Part print with two shaded views. Sizes in mm from the minimum x, y, z corner. A direction names the side the tool comes from. Give positions to 0.01 mm unless a question says otherwise; leave off trailing zeros. Write each loop counter-clockwise with the first axis right and the second up, starting at its lowest first coordinate (ties: lowest second). Pieces come first, ordered by that corner, then holes.
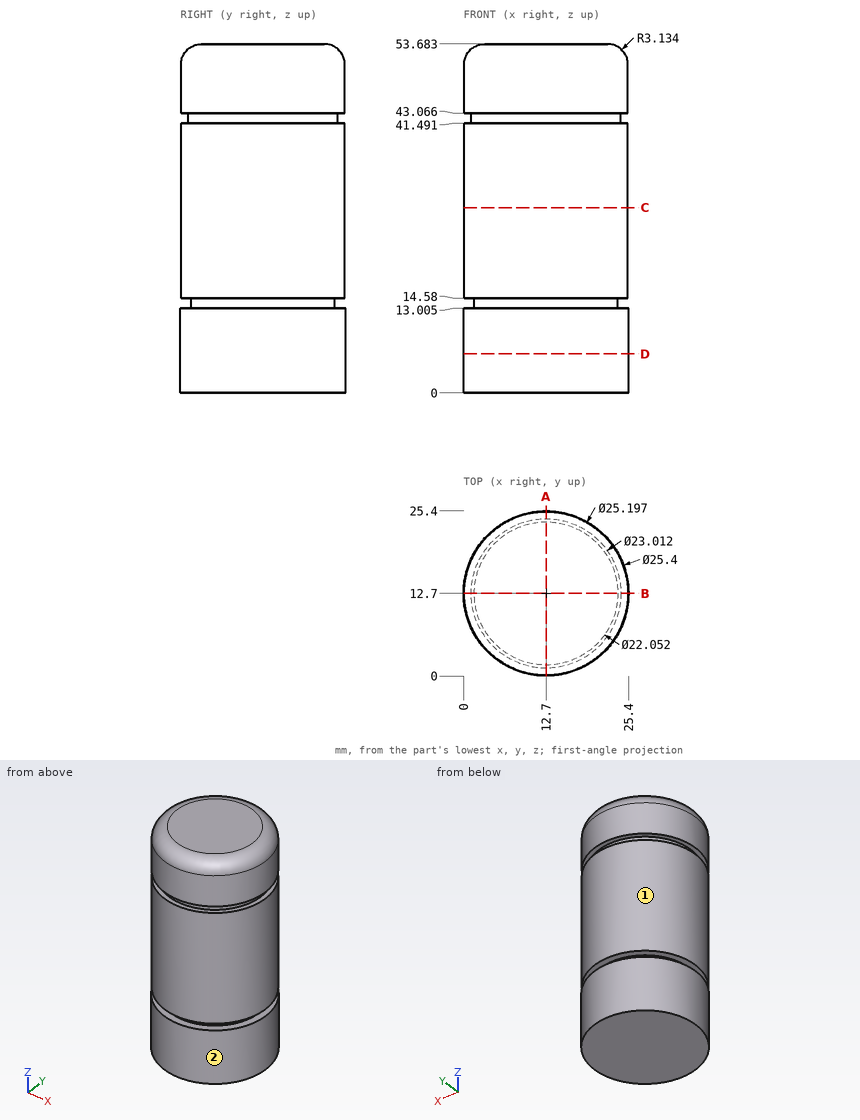
1) Wall check: L1, parallel to Z at x = 22.75, y = 19.5 (1 decimal); L2, parallel to Z at x = 12.5, y = 1 (1 decimal); L3, parallel to Z at x = 21.75, y = 16. Give the ranges that are in metal, low to high.
Answers follow:
L1: z = 0 to 13, 14.6 to 41.5, 43.1 to 52.2
L2: z = 0 to 13, 14.6 to 41.5, 43.1 to 52.7
L3: z = 0 to 53.68
2) Saw through at D-D, the plane z = 6. Write the cut outline in (x, y).
Answers follow:
outline: circle Ø25.4 at (12.7, 12.7)
3) 3-axis set-ups, long thin cutter, end or side, ignore diameter. For the marked faces 1 and 2: which of +Z, -Z, +X, -X, +Y, -Y reach the whole face in a straight line?
Answers follow:
face 1: +Z
face 2: +Z, -Z
4) Pin check, flat tips, straight feed: pin 1 Ø2 at (x, z) = (17.5, 10.5) entering from +Y; pin 2 Ø1.5 at (y, z) = (13.5, 14.5) entering from +X; pin 3 Ø2 at (y, z) = (6, 19.5) entering from +X (1 decimal). Stop position of each tip, or through.
Answers follow:
pin 1: stops at y = 24.82
pin 2: stops at x = 25.3
pin 3: stops at x = 23.9
5) Saw through at A-A, the plane x = 12.7. Write the cut outline in (y, z) (1 decimal).
Answers follow:
outline: (0, 0) - (25.4, 0) - (25.4, 13) - (23.7, 13) - (23.7, 14.6) - (25.3, 14.6) - (25.3, 41.5) - (24.2, 41.5) - (24.2, 43.1) - (25.3, 43.1) - (25.3, 50.5) arc R3.1 ccw to (22.2, 53.7) - (3.2, 53.7) arc R3.1 ccw to (0.1, 50.5) - (0.1, 43.1) - (1.2, 43.1) - (1.2, 41.5) - (0.1, 41.5) - (0.1, 14.6) - (1.7, 14.6) - (1.7, 13) - (0, 13) - close
6) Saw through at C-C, the plane z = 28.5. Write the cut outline in (x, y).
Answers follow:
outline: circle Ø25.2 at (12.7, 12.7)
